Geometry: see drawing. Coordinates: mm, zero at the bounding-box minimum. Coordinates: 2 decimals unless noted, no trailing zeros. Order: outer loops, then holes, each group sorted by start corner. A loop starts at its lowest first (then second) coordinate and runs counter-clockwise, first axis right, second up. Notation, with made-up numbers: (64, -26.75) - (69, -26.75) arc R28 cw to (69, 5.25) - close; hole circle Ø9 at (76, -26). An arc over 180 degrees is marked (long way). Use a Markdown table: item, result. Add a question column.
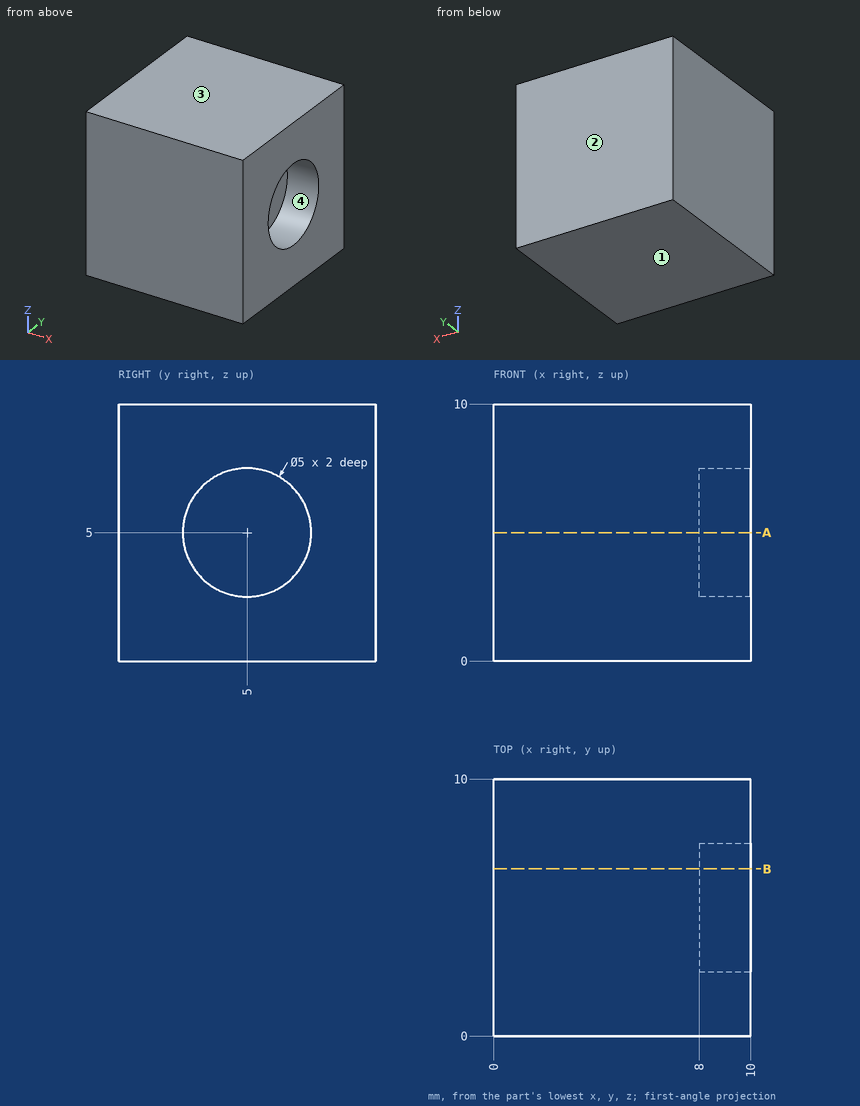
1) Material intervals for L1, parallel to Y at x = 9, z = 5; L2, parallel to X at y = 5.25, z = 4.5, sorted ascending.
2) Cut plane B-B (y = 6.5). Return the cut outline in (x, z).
3) Pull-direction query (Z, two-part tool) for the marked faces 1, 2, 3 and 4; classes: pulls with the +Z half, pulls with the -Z half, needs draft (parallel to the pull), parting line crosses it, or undercut.
4) Contact query for a flat-ended pin moving along its axis: P1, Ø1.5, axis at y = 5, z = 5.5, coming from the +X side. Output: stop coordinate, or through.
5) Cut plane A-A (z = 5). Return the cut outline in (x, y), and give its area (3 significant figures).
Computed:
| question | item | result |
|---|---|---|
| 1 | L1 | y = 0 to 2.5, 7.5 to 10 |
| 1 | L2 | x = 0 to 8 |
| 2 | outline | (0, 0) - (10, 0) - (10, 3) - (8, 3) - (8, 7) - (10, 7) - (10, 10) - (0, 10) - close |
| 3 | face 1 | pulls with the -Z half |
| 3 | face 2 | needs draft |
| 3 | face 3 | pulls with the +Z half |
| 3 | face 4 | undercut |
| 4 | P1 | stops at x = 8 |
| 5 | outline | (0, 0) - (10, 0) - (10, 2.5) - (8, 2.5) - (8, 7.5) - (10, 7.5) - (10, 10) - (0, 10) - close |
| 5 | area | 90.0 mm2 |
